```python
from build123d import *

# Parameters (mm, degrees)
F0_R     = 3.05
F1_DEPTH = 2
F2_W     = 27
F2_H     = 1
F3_DEPTH = 20


with BuildPart() as f1:
    # F0 (on Top) → F1 (new body)
    with BuildSketch(Plane.XY):
        Polygon((6, 20), (6, 0), (28.006723, 0), (28.006723, 9.25), (27.006723, 9.25), (27.006723, 10.55), (54.006723, 10.55), (54.006723, 9.25), (53.006723, 9.25), (53.006723, 0), (74, 0), (74, 20), align=None)
        with Locations((12.5, 10)):
            Circle(F0_R, mode=Mode.SUBTRACT)
        with Locations((67.5, 10)):
            Circle(F0_R, mode=Mode.SUBTRACT)
    extrude(amount=F1_DEPTH)

    # F2 (on face) → F3 (join)
    with BuildSketch(Plane.XY.offset(2)):
        with Locations((40.506723, 11.05)):
            Rectangle(F2_W, F2_H)
        Polygon((27.006723, 9.25), (27.006723, 10.55), (27.006723, 11.55), (26.006723, 11.55), (26.006723, 9.25), align=None)
        Polygon((54.006723, 11.55), (54.006723, 10.55), (54.006723, 9.25), (55.006723, 9.25), (55.006723, 11.55), align=None)
        Polygon((28.006723, 9.25), (27.006723, 9.25), (26.006723, 9.25), (26.006723, 8.25), (28.006723, 8.25), align=None)
        Polygon((55.006723, 9.25), (54.006723, 9.25), (53.006723, 9.25), (53.006723, 8.25), (55.006723, 8.25), align=None)
    extrude(amount=F3_DEPTH)


solid = f1.part
```
Source: CAD feature listing. Evaluate the final solid. Frame: model axes, mm. A direction names the side the tool comes from. Coordinates: 2 decimals unless noted, no trailing zeros. Order: outer loops, then holes, each group sorted by start corner. A loop starts at its lowest first (then second) coordinate and runs counter-clockwise, first axis right, second up. Notation, with made-up numbers: M 82,-28 L 89,-28 A36 ccw 89,11 Z; hole C -23.5,-28 d6. An arc over 180 degrees is marked long. Write each question's results on one line, items separated by ' | '. Start each with the question number.
1) Section query D-D (x = 40). Return the cut outline in (y, z), plus the area to 3 significant figures.
2) Line query: line 1 (Y direction, x = 67.5, z = 0.85); line 2 (X direction, y = 9.75, z = 13.5); line 3 (Z direction, x = 62.5, y = 15). Output: solid intervals per line, ascending. Write a range as from..to.
3) Draft query along X for faces 4 (the face through (27, 8.25, 12)), 5 (the face through (55.007, 10, 12)), 6 (the face through (40, 10.55, 11)). Return one class per face: released by +X, released by -X, zero draft, split by the parting line, or undercut.
4) Section query C-C (z = 14.25). Return the cut outline in (x, y), plus the area to 3 significant figures.
5) Section query A-A (x = 12.5). Return the cut outline in (y, z).
6) Section query B-B (y = 3.25). Return the cut outline in (x, z).
7) Access query for faces 1 (the face through (54.007, 10, 11)), 2 (the face through (53.007, 8.4, 6.1)), 3 (the face through (41, 11.55, 12)). Directions: +Z, -Z, +X, -X, +Y, -Y. A direction counts if a zero-diameter tool reaches every point of the face in a straight line with its end or side. Return the directions, or none.
8) Contact query for flat-ended pins moving along their axis: pin 1 Ø5 at (x, z) = (54.5, 14.5) entering from -Y; pin 2 Ø10 at (x, z) = (43, 13) entering from +Y; pin 3 Ø1 at (y, z) = (9.5, 12) entering from -X; pin 4 Ø7.5 at (y, z) = (3.5, 6.5) entering from -X. Output: stop coordinate, or through.
Answers:
1) outline: M 10.55,0 L 20,0 L 20,2 L 11.55,2 L 11.55,22 L 10.55,22 Z | area: 38.9 mm^2
2) line 1: y = 0..6.95, 13.05..20 | line 2: x = 26.01..27.01, 54.01..55.01 | line 3: z = 0..2
3) face 4: zero draft | face 5: released by +X | face 6: undercut
4) outline: M 26.01,8.25 L 28.01,8.25 L 28.01,9.25 L 27.01,9.25 L 27.01,10.55 L 54.01,10.55 L 54.01,9.25 L 53.01,9.25 L 53.01,8.25 L 55.01,8.25 L 55.01,11.55 L 26.01,11.55 Z | area: 35.6 mm^2
5) outline: M 0,0 L 6.95,0 L 6.95,2 L 0,2 Z; M 13.05,0 L 20,0 L 20,2 L 13.05,2 Z
6) outline: M 6,0 L 28.01,0 L 28.01,2 L 6,2 Z; M 53.01,0 L 74,0 L 74,2 L 53.01,2 Z
7) face 1: +Z, -Z | face 2: +Z, -Z, -Y | face 3: +Z, +X, -X, +Y
8) pin 1: stops at y = 8.25 | pin 2: stops at y = 11.55 | pin 3: stops at x = 26.01 | pin 4: passes through
